Design review of the part built by this model. Coordinates are the model's own, in mm. Face numbers are marked on the shaded views. A direction names the side the tool comes from. Coordinates: 2 decimals unless noted, no trailing zeros. Loops run counter-clockwise (first coordinate to the right, second up) from the corner with the lowest first, then second, coordinate; pieces in that order, holes last. Notation, with made-up numbers: (-36.75, 50) -> (20.25, 50) arc R22 ccw to (20.25, 70) -> close; hole circle Ø1 at (-35, 75). An arc over 180 degrees is marked (long way). Use one line per item in the form item = value. Start each with the question number.
1. Consider section A-A (x = 31.75). State the section outline as (y, z) points, then the cut area to 3 significant figures.
2. Consider section B-B (y = -12.7). State the section outline as (x, z) points.
3. For pin 1 (5 mm diameter, centred on x = 31.75, y = -12.7, fed in from -Z); pin 2 (2 mm diameter, centred on y = 36, z = 8.5, fed in from -X); pin 3 (6 mm diameter, centred on x = -13.5, z = 6.5, fed in from -Y); pin 4 (2 mm diameter, centred on x = -9, z = 7.5, fed in from +Y), all flat-tipped, find the tip position at first contact; note any pin that passes through.
4. Consider section D-D (x = 8.25). State the section outline as (y, z) points.
5. Wall thickness on line 1 (Y direction, x = 20, z = 3.25); line 2 (Y direction, x = 7.5, z = 6); line 3 (X direction, y = -15.5, z = 4): over which ranges is each line inside the solid? List them lowest first. Write a range as from..to.
6. The part is to be moulded in two halves that separate along X. For the marked faces 1, 2 and 3, say which applies: released by +X, released by -X, zero draft, split by the parting line, or undercut.
7. Machinability: for the marked faces 4, 5 and 6, which of the approach directions +Z, -Z, +X, -X, +Y, -Y give a long, thin tool a straight path to every point of the face, cutting with its end or side? Answer none if there is none.
8. Consider section C-C (z = 1.25). State the section outline as (x, y) points.
from build123d import *

# Parameters (mm, degrees)
SKETCH1_R           = 2.75
BOSS_EXTRUDE1_DEPTH = 10
FILLET1_R           = 5
FILLET2_R           = 2


with BuildPart() as part:
    # Sketch1 → Boss-Extrude1 (new body)
    with BuildSketch(Plane.XY):
        Polygon((-60, 10), (11.568542495, 81.568542495), (40, 81.568542495), (40, -25.4), (0, -25.4), (0, 0), (-60, 0), align=None)
        with Locations((8.25, -12.7)):
            Circle(SKETCH1_R, mode=Mode.SUBTRACT)
        with Locations((20, -12.7)):
            Circle(SKETCH1_R, mode=Mode.SUBTRACT)
        with Locations((31.75, -12.7)):
            Circle(SKETCH1_R, mode=Mode.SUBTRACT)
        with BuildLine():
            Line((17.781745931, 66.568542495), (25, 66.568542495))
            Line((25, 66.568542495), (25, 10))
            Line((25, 10), (-38.786796564, 10))
            ThreePointArc((-38.786796564, 10), (-7.645233685, 35.426979616), (17.781745931, 66.568542495))
        make_face(mode=Mode.SUBTRACT)
    extrude(amount=BOSS_EXTRUDE1_DEPTH)

    # Fillet1
    # the kernel refuses this fillet: 5 mm, written as the material it adds along each edge
    with BuildSketch(Plane(origin=(17.781745931, 66.568542495, 0), x_dir=(-0.556881790774907, -0.8305917595927212, 0), z_dir=(0, 0, 1))) as fillet1_piece_1:
        with BuildLine():
            CenterArc((2.667557701, 4.999891542), FILLET1_R, 213.840425913, 55.782189142)
            Line((-1.485401097, 2.215482588), (0, 0))
            ThreePointArc((0, 0), (1.317312445, 0.004338327), (2.63462489, 0))
        make_face()
    extrude(amount=10)
    with BuildSketch(Plane(origin=(25, 66.568542495, 0), x_dir=(0, -1, 0), z_dir=(0, 0, 1)), Plane(origin=(25, 10, 0), x_dir=(-1, 0, 0), z_dir=(0, 0, 1)), Plane(origin=(0, 0, 0), x_dir=(0, -1, 0), z_dir=(0, 0, 1))) as fillet1_piece_2:
        with BuildLine():
            CenterArc((FILLET1_R, -FILLET1_R), FILLET1_R, 90, 90)
            Line((0, -FILLET1_R), (0, 0))
            Line((0, 0), (FILLET1_R, 0))
        make_face()
    extrude(amount=10)
    # the kernel refuses this fillet: 5 mm, written as the material it takes off along each edge
    with BuildSketch(Plane(origin=(-60, 0, -12.5), x_dir=(0, 1, 0), z_dir=(0, 0, 1))) as fillet1_2_piece_1:
        with BuildLine():
            CenterArc((FILLET1_R, -FILLET1_R), FILLET1_R, 90, 90)
            Line((0, -FILLET1_R), (0, 0))
            Line((0, 0), (FILLET1_R, 0))
        make_face()
    extrude(amount=35, mode=Mode.SUBTRACT)
    with BuildSketch(Plane(origin=(-60, 10, -5.17766953), x_dir=(0.7071067811865476, 0.7071067811865476, 0), z_dir=(0, 0, 1))) as fillet1_2_piece_2:
        with BuildLine():
            CenterArc((FILLET1_R * 0.414213562373, -FILLET1_R), FILLET1_R, 90, 45)
            Line((-FILLET1_R * 0.292893218813, -FILLET1_R * 0.292893218813), (0, 0))
            Line((0, 0), (FILLET1_R * 0.414213562373, 0))
        make_face()
    extrude(amount=20.355339059, mode=Mode.SUBTRACT)
    with BuildSketch(Plane(origin=(0, -25.4, -12.5), x_dir=(1, 0, 0), z_dir=(0, 0, 1)), Plane(origin=(40, -25.4, -12.5), x_dir=(0, 1, 0), z_dir=(0, 0, 1)), Plane(origin=(40, 81.568542495, -12.5), x_dir=(-1, 0, 0), z_dir=(0, 0, 1))) as fillet1_2_piece_3:
        with BuildLine():
            CenterArc((FILLET1_R, FILLET1_R), FILLET1_R, 180, 90)
            Line((0, FILLET1_R), (0, 0))
            Line((0, 0), (FILLET1_R, 0))
        make_face()
    extrude(amount=35, mode=Mode.SUBTRACT)
    with BuildSketch(Plane(origin=(11.568542495, 81.568542495, -5.17766953), x_dir=(-0.7071067811865509, -0.707106781186544, 0), z_dir=(0, 0, 1))) as fillet1_2_piece_4:
        with BuildLine():
            CenterArc((FILLET1_R * 0.414213562373, FILLET1_R), FILLET1_R, 225, 45)
            Line((-FILLET1_R * 0.292893218813, FILLET1_R * 0.292893218813), (0, 0))
            Line((0, 0), (FILLET1_R * 0.414213562373, 0))
        make_face()
    extrude(amount=20.355339059, mode=Mode.SUBTRACT)

    # Fillet2
    fillet2_edges = [part.edges().sort_by_distance(p)[0] for p in [
        (-38.786796564, 10, 5),
    ]]
    fillet(fillet2_edges, radius=FILLET2_R)


solid = part.part
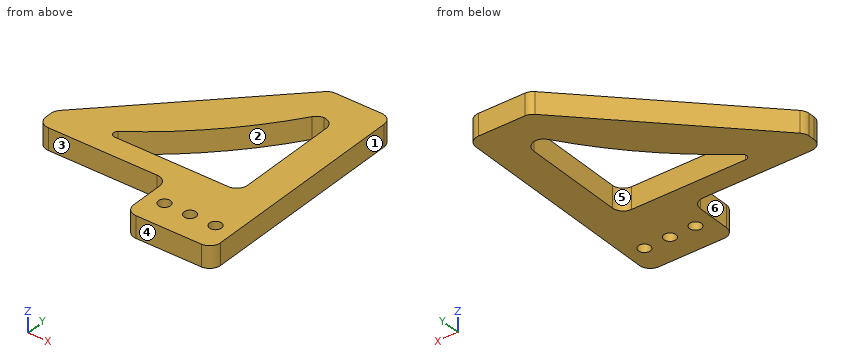
Geometry check:
q1.outline = (-25.4, 0) -> (-15.45, 0) -> (-15.45, 10) -> (-25.4, 10) -> close; (-9.95, 0) -> (81.57, 0) -> (81.57, 10) -> (-9.95, 10) -> close
q1.area = 1,010 mm²
q2.outline = (0, 0) -> (5.5, 0) -> (5.5, 10) -> (0, 10) -> close; (11, 0) -> (17.25, 0) -> (17.25, 10) -> (11, 10) -> close; (22.75, 0) -> (29, 0) -> (29, 10) -> (22.75, 10) -> close; (34.5, 0) -> (40, 0) -> (40, 10) -> (34.5, 10) -> close
q3.pin_1 = through
q3.pin_2 = -35
q3.pin_3 = 0
q3.pin_4 = 62
q4.outline = (-25.4, 0) -> (-15.45, 0) -> (-15.45, 10) -> (-25.4, 10) -> close; (-9.95, 0) -> (10, 0) -> (10, 10) -> (-9.95, 10) -> close; (53.35, 0) -> (78.25, 0) -> (78.25, 10) -> (53.35, 10) -> close
q5.line_1 = -25.4..-15.45, -9.95..10, 66.55..81.57
q5.line_2 = -25.4..-15.35, -10.05..10, 52.4..77.5
q5.line_3 = 0..40
q6.face_1 = released by +X
q6.face_2 = undercut
q6.face_3 = zero draft
q7.face_4 = +Z, -Z, +X, -X, -Y
q7.face_5 = +Z, -Z
q7.face_6 = +Z, -Z, -X, -Y
q8.outline = (-60, 5) arc R5 ccw to (-55, 0) -> (-5, 0) arc R5 cw to (0, -5) -> (0, -20.4) arc R5 ccw to (5, -25.4) -> (35, -25.4) arc R5 ccw to (40, -20.4) -> (40, 76.57) arc R5 ccw to (35, 81.57) -> (13.64, 81.57) arc R5 ccw to (10.1, 80.1) -> (-58.54, 11.46) arc R5 ccw to (-60, 7.93) -> close; hole (-33.48, 13.63) arc R2 ccw to (-32.32, 10) -> (20, 10) arc R5 ccw to (25, 15) -> (25, 61.57) arc R5 ccw to (20.22, 66.56) arc R5 ccw to (16.31, 64.38) arc R200 cw to start; hole circle Ø5.5 at (8.25, -12.7); hole circle Ø5.5 at (20, -12.7); hole circle Ø5.5 at (31.75, -12.7)
